```python
from build123d import *

# Parameters (mm, degrees)
F1_DEPTH  = 5
F2_ANGLE  = 30
F4_COUNT  = 6
F5_R      = 30
F6_DEPTH  = 12.5
F11_DEPTH = 4.1938354
F12_R     = 15
F13_DEPTH = 12.5


# Not quite as in the source:
# - an extrude ends at something that could not be found from the text; its depth is read off the source's solid
# - a feature of the source that left no trace in its solid (it failed there, or was rolled back) is left out
# - a pattern or mirror of a feature is missing from the dataset's text; its kind, count and spacing are read off the source's solid


with BuildPart() as f1:
    # F0 (on Top) → F1 (new body, symmetric)
    with BuildSketch(Plane.XY):
        with BuildLine():
            Line((96.5925826289, 25.8819045103), (0, 0))
            Line((0, 0), (96.5925826289, -25.8819045103))
            ThreePointArc((96.5925826289, -25.8819045103), (100, 0), (96.5925826289, 25.8819045103))
        make_face()
    extrude(amount=F1_DEPTH, both=True)


with BuildPart() as f1_1:
    # F2: moved
    add(f1.part.rotate(Axis((70.1462253928, 0, 0), (1, 0, 0)), F2_ANGLE))


with BuildPart() as f4_1:
    # F4: instance of F1
    add(f1_1.part.rotate(Axis((0, 0, 33.6874611676), (0, 0, 1)), 1 * 360 / F4_COUNT))


with BuildPart() as f4_2:
    # F4: instance of F1
    add(f1_1.part.rotate(Axis((0, 0, 33.6874611676), (0, 0, 1)), 2 * 360 / F4_COUNT))


with BuildPart() as f4_3:
    # F4: instance of F1
    add(f1_1.part.rotate(Axis((0, 0, 33.6874611676), (0, 0, 1)), 3 * 360 / F4_COUNT))


with BuildPart() as f4_4:
    # F4: instance of F1
    add(f1_1.part.rotate(Axis((0, 0, 33.6874611676), (0, 0, 1)), 4 * 360 / F4_COUNT))


with BuildPart() as f4_5:
    # F4: instance of F1
    add(f1_1.part.rotate(Axis((0, 0, 33.6874611676), (0, 0, 1)), 5 * 360 / F4_COUNT))


with BuildPart() as f1_2:
    add(f1_1.part)

    add(f4_1.part)  # F6 merges F4_1

    add(f4_2.part)  # F6 merges F4_2

    add(f4_3.part)  # F6 merges F4_3

    add(f4_4.part)  # F6 merges F4_4

    add(f4_5.part)  # F6 merges F4_5
    # F5 (on Top) → F6 (join, symmetric)
    with BuildSketch(Plane.XY):
        Circle(F5_R)
    extrude(amount=F6_DEPTH, both=True)

    # F11 (cut, through all): a face of the model
    f11_faces = [f1_2.faces().sort_by_distance(p)[0] for p in [
        (0, 0, -12.5),
    ]]
    f11 = extrude(f11_faces, amount=-F11_DEPTH, mode=Mode.SUBTRACT)

    # F11_copies: F11 across plane
    add(f11.mirror(Plane.XY), mode=Mode.SUBTRACT)

    # F12 (on Top) → F13 (cut, symmetric)
    with BuildSketch(Plane.XY):
        Circle(F12_R)
    extrude(amount=F13_DEPTH, both=True, mode=Mode.SUBTRACT)


solid = f1_2.part
```
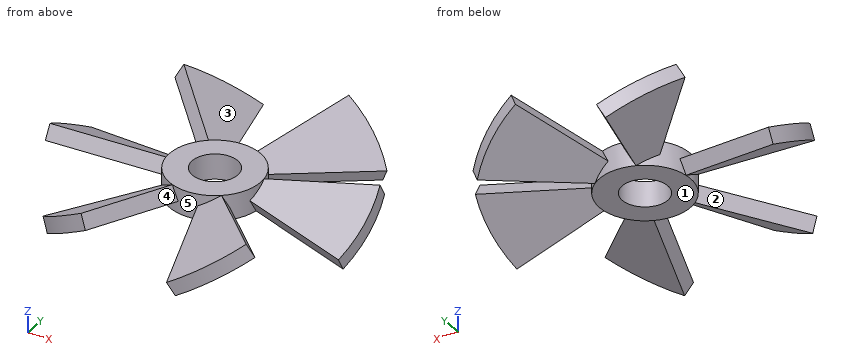
Verification items for the finished model (mm, model axes). Face numbers are marked on the shaded views. A direction names the side the tool comes from. Coordinates: 2 decimals unless noted, no trailing zeros. Loops run counter-clockwise (first coordinate to the right, second up) from the corner with the lowest first, then second, coordinate; pieces in that order, holes last. Notation, with made-up numbers: (83, 59) -> (123, 59) arc R10 cw to (123, 75) -> close; hole circle Ø3 at (42, 18.5). An arc over 180 degrees is marked (long way). Answer in a Markdown table with one row per item.
1) Section check C-C (z = -13). Give the number of separate pieces and of enclosed holes in the cut face, and give its area (3 significant figures).
The answers:
| item | result |
|---|---|
| separate pieces | 6 |
| enclosed holes | 0 |
| area | 1,000 mm2 |
2) Section check A-A (x = 0). Record the cut outline in (y, z), and give its area (3 significant figures).
The answers:
| item | result |
|---|---|
| outline | (-30, -8.31) -> (-15, -8.31) -> (-15, 8.31) -> (-30, 8.31) -> close; (15, -8.31) -> (30, -8.31) -> (30, 8.31) -> (15, 8.31) -> close |
| area | 498 mm2 |
3) Depth check by flat-ended pin: P1, Ø1.5, axis at x = -62.5, z = -11, coming from the +Y side; P2, Ø3, axis at x = -37.5, y = -3, coming from the +Z side; P3, Ø1, axis at y = -56, z = -12.5, coming from the +X side. Enter the tip coordinate at first touch or a pass-through.
The answers:
| item | result |
|---|---|
| P1 | stops at y = 13.48 |
| P2 | stops at z = 8.37 |
| P3 | stops at x = 19.92 |
4) Section check B-B (y = -61). Record the cut outline in (x, z), and give its area (3 significant figures).
The answers:
| item | result |
|---|---|
| outline | (-60.34, -6.79) -> (-53.68, -15) -> (-16.03, 3.82) -> (-21.12, 12.82) -> close; (16.03, -3.82) -> (21.12, -12.82) -> (60.34, 6.79) -> (53.68, 15) -> close |
| area | 888 mm2 |
5) Access from +Z, -Z, +X, -X, +Y, -Y to the whole of each face (thin tool, end or side, straight path). Record for the marked faces 1, 2, 3, 4 and 5.
The answers:
| item | result |
|---|---|
| face 1 | -Z |
| face 2 | -Z, -X |
| face 3 | +Z, +Y |
| face 4 | +Z, -Y |
| face 5 | -Y |
6) Scan lines: line 1 along Y through (x, z) = (0, 0); line 2 along Z through (x, y) = (-14, 11.5); line 3 along X through (y, z) = (64, -1). Record each from-to range of solid material in increasing order. Write a range as from..to.
The answers:
| item | result |
|---|---|
| line 1 | y = -30..-15, 15..30 |
| line 2 | z = -8.31..8.31 |
| line 3 | x = -46.5..-23.4, 27.4..50.5 |
